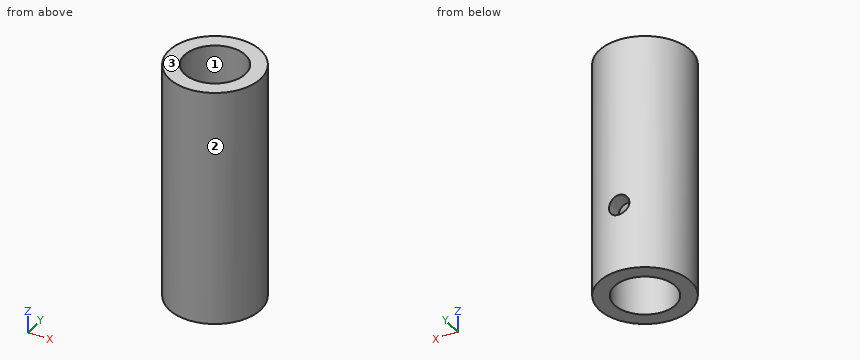
Autodesk Inventor part; units mm, degrees
ref_plane "Work Plane1" through (0, 6.75, 0) normal (0, 1, 0) x (-1, 0, 0)
ref_plane "YZ Plane" through (0, 0, 0) normal (1, 0, 0) x (0, 1, 0)
ref_plane "XY Plane" through (0, 0, 0) normal (0, 0, 1) x (1, 0, 0)
sketch "Sketch1" plane through (0, 0, 0) normal (0, 0, 1) x (1, 0, 0)
  circle A0 centre (0, 0) radius 6.75
  dimension "d0" = 13.5
extrude "Extrusion1" add sketch "Sketch1" along normal blind 35
sketch "Sketch2" plane through (0, 0, 35) normal (0, 0, 1) x (1, 0, 0)
  point P0 (0, 0)
hole "Hole1" at (0, 0, 35) direction (0, 0, -1) diameter 9 end through all
ref_plane "Work Plane1" through (0, 6.75, 0) normal (0, 1, 0) x (-1, 0, 0)
sketch "Sketch3" plane through (0, 6.75, 0) normal (0, 1, 0) x (-1, 0, 0)
  line L0 (6.75, 0) -> (-6.75, 0)
  point P0 (0, 0)
  point P1 (0, 10)
  dimension "d10" = 10
  dimension "d11" = 6.75
hole "Hole2" at (0, 6.75, 10) direction (0, -1, 0) diameter 3 end up to surface
properties part number "HUDSON-1-74"
Part model, mm, in its own coordinate system. Face numbers are marked on the shaded views. Coordinates: 2 decimals unless noted, no trailing zeros. Order: outer loops, then holes, each group sorted by start corner. A loop starts at its lowest first (then second) coordinate and runs counter-clockwise, first axis right, second up. Notation, with made-up numbers: (24, 81) - (75, 81) arc R22 ccw to (75, 87) - close; hole circle Ø9 at (34, -27). An arc over 180 degrees is marked (long way). Return JSON: item names as keys, results as strings. Group by question number.
Item 1: Cut at D-D (x = 3). List the corners of the cut face in (y, z), plus the area to 3 significant figures.
Item 2: Drill centre lines: probe 1 along Y at (x, z) = (0, 13); probe 2 along Z at (x, y) = (0, 6); probe 3 along X at (y, z) = (-1.75, 22.5). Where is each one in solid material? Low to high. Write a range as from..to.
Item 3: Pin check, flat tip, straight feed: pin 1 (1.5 mm diameter, centred on x = 5, z = 14, fed in from -Y). Stop position of the tip, or through.
Item 4: Pull direction X, two halves, no side cores. Call the marked faces 1, 2 and 3: pulls with the +X half, pulls with the -X half, needs draft (parallel to the pull), parting line crosses it, or undercut.
Item 5: Cut at B-B (y = 2.75). List the corners of the cut face in (x, z), plus the area to 3 significant figures.
Item 6: Cut at C-C (z = 26.5). List the corners of the cut face in (x, y), plus the area to 3 significant figures.
Item 7: Cut at A-A (x = 0). List the corners of the cut face in (y, z).
Check values:
{
 "1": {"outline": "(-6.05, 0) - (-3.35, 0) - (-3.35, 35) - (-6.05, 35) - close; (3.35, 0) - (6.05, 0) - (6.05, 35) - (3.35, 35) - close", "area": "188 mm2"},
 "2": {"probe 1": "y = -6.75..-4.5, 4.5..6.75", "probe 2": "z = 0..8.5, 11.5..35", "probe 3": "x = -6.52..-4.15, 4.15..6.52"},
 "3": {"pin 1": "stops at y = -5.24"},
 "4": {"face 1": "undercut", "face 2": "parting line crosses it", "face 3": "needs draft"},
 "5": {"outline": "(-6.16, 0) - (-3.56, 0) - (-3.56, 35) - (-6.16, 35) - close; (3.56, 0) - (6.16, 0) - (6.16, 35) - (3.56, 35) - close", "area": "182 mm2"},
 "6": {"outline": "circle Ø13.5 at (0, 0); hole circle Ø9 at (0, 0)", "area": "79.5 mm2"},
 "7": {"outline": "(-6.75, 0) - (-4.5, 0) - (-4.5, 35) - (-6.75, 35) - close; (4.5, 0) - (6.75, 0) - (6.75, 8.5) - (4.5, 8.5) - close; (4.5, 11.5) - (6.75, 11.5) - (6.75, 35) - (4.5, 35) - close"}
}
